For this review, take the finished solid that the model builds, in its own axes (mm). A direction names the side the tool comes from. Round coordinates to 2 decimals unless told otherwise and drop trailing zeros. Order: outer loops, then holes, each group sorted by start corner. A loop starts at its lowest first (then second) coordinate and runs counter-clockwise, first axis right, second up. Notation, with made-up numbers: M 25.5,32.25 L 64.5,32.25 A23 ccw 64.5,40.25 Z; hole C -10.75,83.25 d3. An arc over 180 degrees is marked long. Answer in a Markdown table with one row per item. Add a question column.
```python
from build123d import *

# Parameters (mm, degrees)
SKETCH_1_W          = 54
SKETCH_1_H          = 40
SKETCH_1_R          = 1.6
SKETCH_1_W_2        = 80.56
SKETCH_1_H_2        = 100
EXTRUDE_1_DEPTH     = 5
CUT_EXTRUDE_5_DEPTH = 99.729318847
FILLET_1_R          = 5


with BuildPart() as part:
    # 草图1 → 凸台-拉伸1 (new body)
    # profile 1 of 2: a face of its own
    with BuildSketch(Plane(origin=(0, 0, 0), x_dir=(1, 0, 0), z_dir=(0, 1, 0))):
        with Locations((0, -70)):
            Rectangle(SKETCH_1_W, SKETCH_1_H)
        with Locations(Location((-14, -70, 0), (0, 0, 270))):
            Circle(SKETCH_1_R, mode=Mode.SUBTRACT)
        with Locations(Location((14, -70, 0), (0, 0, 270))):
            Circle(SKETCH_1_R, mode=Mode.SUBTRACT)
    # profile 2 of 2: a face of its own
    with BuildSketch(Plane(origin=(0, 0, 0), x_dir=(1, 0, 0), z_dir=(0, 1, 0))):
        Rectangle(SKETCH_1_W_2, SKETCH_1_H_2)
        with Locations(Location((15.25, 15.25, 0), (0, 0, 270))):
            Circle(SKETCH_1_R, mode=Mode.SUBTRACT)
        with Locations(Location((-15.25, 15.25, 0), (0, 0, 270))):
            Circle(SKETCH_1_R, mode=Mode.SUBTRACT)
        with Locations(Location((-34.12, -40.19, 0), (0, 0, 270))):
            Circle(SKETCH_1_R, mode=Mode.SUBTRACT)
        with Locations(Location((15.09, -40.19, 0), (0, 0, 270))):
            Circle(SKETCH_1_R, mode=Mode.SUBTRACT)
        with Locations(Location((15.09, 46.89, 0), (0, 0, 270))):
            Circle(SKETCH_1_R, mode=Mode.SUBTRACT)
        with Locations(Location((-34.12, 46.89, 0), (0, 0, 270))):
            Circle(SKETCH_1_R, mode=Mode.SUBTRACT)
        with Locations(Location((15.25, -15.25, 0), (0, 0, 270))):
            Circle(SKETCH_1_R, mode=Mode.SUBTRACT)
        with Locations(Location((-15.25, -15.25, 0), (0, 0, 270))):
            Circle(SKETCH_1_R, mode=Mode.SUBTRACT)
    extrude(amount=EXTRUDE_1_DEPTH)

    # 草图7 → 切除-拉伸5 (cut, through all)
    with BuildSketch(Plane(origin=(0, 0, 0), x_dir=(1, 0, 0), z_dir=(0, 1, 0))):
        with BuildLine():
            ThreePointArc((-6.01040764, -10.960155108), (-6.01040764, -13.788582233), (-8.838834765, -13.788582233))
            Line((-8.838834765, -13.788582233), (-13.788582233, -8.838834765))
            ThreePointArc((-13.788582233, -8.838834765), (-13.788582233, -6.01040764), (-10.960155108, -6.01040764))
            Line((-10.960155108, -6.01040764), (-6.01040764, -10.960155108))
        make_face()
        with BuildLine():
            ThreePointArc((2.121320344, -9.192388155), (2.121320344, -12.02081528), (-0.707106781, -12.02081528))
            Line((-0.707106781, -12.02081528), (-12.02081528, -0.707106781))
            ThreePointArc((-12.02081528, -0.707106781), (-12.02081528, 2.121320344), (-9.192388155, 2.121320344))
            Line((-9.192388155, 2.121320344), (2.121320344, -9.192388155))
        make_face()
        with BuildLine():
            Line((-10.253048327, 7.424621202), (7.424621202, -10.253048327))
            ThreePointArc((7.424621202, -10.253048327), (10.253048327, -10.253048327), (10.253048327, -7.424621202))
            Line((10.253048327, -7.424621202), (-7.424621202, 10.253048327))
            ThreePointArc((-7.424621202, 10.253048327), (-10.253048327, 10.253048327), (-10.253048327, 7.424621202))
        make_face()
        with BuildLine():
            Line((-2.121320344, 9.192388155), (9.192388155, -2.121320344))
            ThreePointArc((9.192388155, -2.121320344), (12.02081528, -2.121320344), (12.02081528, 0.707106781))
            Line((12.02081528, 0.707106781), (0.707106781, 12.02081528))
            ThreePointArc((0.707106781, 12.02081528), (-2.121320344, 12.02081528), (-2.121320344, 9.192388155))
        make_face()
        with BuildLine():
            Line((6.01040764, 10.960155108), (10.960155108, 6.01040764))
            ThreePointArc((10.960155108, 6.01040764), (13.788582233, 6.01040764), (13.788582233, 8.838834765))
            Line((13.788582233, 8.838834765), (8.838834765, 13.788582233))
            ThreePointArc((8.838834765, 13.788582233), (6.01040764, 13.788582233), (6.01040764, 10.960155108))
        make_face()
        with BuildLine():
            ThreePointArc((-23.25, 12.5), (-25.25, 10.5), (-27.25, 12.5))
            Line((-27.25, 12.5), (-27.25, 37.5))
            ThreePointArc((-27.25, 37.5), (-25.25, 39.5), (-23.25, 37.5))
            Line((-23.25, 37.5), (-23.25, 12.5))
        make_face()
        with BuildLine():
            Line((23.25, 37.5), (23.25, 12.5))
            ThreePointArc((23.25, 12.5), (25.25, 10.5), (27.25, 12.5))
            Line((27.25, 12.5), (27.25, 37.5))
            ThreePointArc((27.25, 37.5), (25.25, 39.5), (23.25, 37.5))
        make_face()
        with BuildLine():
            Line((-23.25, -37.5), (-23.25, -12.5))
            ThreePointArc((-23.25, -12.5), (-25.25, -10.5), (-27.25, -12.5))
            Line((-27.25, -12.5), (-27.25, -37.5))
            ThreePointArc((-27.25, -37.5), (-25.25, -39.5), (-23.25, -37.5))
        make_face()
        with BuildLine():
            ThreePointArc((23.25, -12.5), (25.25, -10.5), (27.25, -12.5))
            Line((27.25, -12.5), (27.25, -37.5))
            ThreePointArc((27.25, -37.5), (25.25, -39.5), (23.25, -37.5))
            Line((23.25, -37.5), (23.25, -12.5))
        make_face()
        with BuildLine():
            Line((-9, -55), (9, -55))
            ThreePointArc((9, -55), (14, -50), (9, -45))
            Line((9, -45), (-9, -45))
            ThreePointArc((-9, -45), (-14, -50), (-9, -55))
        make_face()
    extrude(amount=CUT_EXTRUDE_5_DEPTH, mode=Mode.SUBTRACT)

    # 圆角1
    fillet_1_edges = [part.edges().sort_by_distance(p)[0] for p in [
        (-40.28, 2.5, 50),
        (-40.28, 2.5, -50),
        (40.28, 2.5, -50),
        (40.28, 2.5, 50),
        (27, 2.5, 90),
        (-27, 2.5, 90),
    ]]
    fillet(fillet_1_edges, radius=FILLET_1_R)


solid = part.part
```
1. To check wall thickness, follow probe 1 along X at (y, z) = (4.5, 22); probe 2 along X at (y, z) = (1.4, -15); probe 3 along X at (y, z) = (2.2, 40.19). State the ranges of each line that lie inside material, in increasing order. Write a range as [from, to].
2. The part is to be moulded in two halves that separate along X. For faces 1 (the cylindrical face through (2.15, 2.46, 11.99)), 2 (the cylindrical face through (38.85, 2.54, 48.5)), 3 (the flat face through (-1, 0, 19)), 4 (the cylindrical face through (-12.05, 2.46, -2.09)), say which applies: pulls with the +X half, pulls with the -X half, needs draft (parallel to the pull), parting line crosses it, or undercut.
3. Consider section D-D on z = 61.5. Write out the cut boundary in (x, y).
4. Clearance check with a flat-ended pin moving along its axis: pin 1 Ø1.5 at (y, z) = (3.5, 65.5) entering from -X. State where the tip first meets the part, or that it passes through.
5. For faces 5 (the flat face through (-11.28, 2.46, 11.35)), 6 (the cylindrical face through (38.78, 2.54, -48.57)), list the 3-axis set-ups (+Z, -Z, +X, -X, +Y, -Y) from which the entire face can be reached by the end or side of a thin tool; tool diameter is ignored.
6. Consider section B-B on x = -25.25. Write out the cut boundary in (y, z).
7. Consider section C-C on y = 2.3. State how many separate pieces and enclosed holes the cut face has, plus the area to 3 significant figures.
8. Consider section A-A on z = -33. Write out the cut boundary in (x, y).
Solved:
| question | item | result |
|---|---|---|
| 1 | probe 1 | x = [-40.28, -27.25], [-23.25, 23.25], [27.25, 40.28] |
| 1 | probe 2 | x = [-40.28, -27.25], [-23.25, -16.83], [-13.67, 13.67], [16.83, 23.25], [27.25, 40.28] |
| 1 | probe 3 | x = [-40.28, -35.72], [-32.52, 13.49], [16.69, 40.28] |
| 2 | face 1 | undercut |
| 2 | face 2 | pulls with the +X half |
| 2 | face 3 | needs draft |
| 2 | face 4 | undercut |
| 3 | outline | M -27,0 L 27,0 L 27,5 L -27,5 Z |
| 4 | pin 1 | stops at x = -27 |
| 5 | face 5 | +Y, -Y |
| 5 | face 6 | -Z, +X, +Y, -Y |
| 6 | outline | M 0,-50 L 5,-50 L 5,-39.5 L 0,-39.5 Z; M 0,-10.5 L 5,-10.5 L 5,10.5 L 0,10.5 Z; M 0,39.5 L 5,39.5 L 5,88.8 L 0,88.8 Z |
| 7 | separate pieces | 1 |
| 7 | enclosed holes | 20 |
| 7 | area | 9,050 mm^2 |
| 8 | outline | M -40.28,0 L -27.25,0 L -27.25,5 L -40.28,5 Z; M -23.25,0 L 23.25,0 L 23.25,5 L -23.25,5 Z; M 27.25,0 L 40.28,0 L 40.28,5 L 27.25,5 Z |
